Autodesk Fusion 360 part; units mm, degrees
sketch "Sketch1" plane through (0, 0, 0) normal (0, 1, 0) x (1, 0, 0) in component "SwitchSpacer"
  arc A0 (-5.8311, -8.732) -> (-5.8573, 8.7145) centre (0, 0) cw
  arc A1 (-4.6183, -9.4298) -> (-5.8311, -8.732) centre (-5.2363, -9.1011) cw
  line L0 (-20, 3.982) -> (0, 3.982)
  arc A2 (10.4756, 0.7154) -> (10.4777, -0.6839) centre (10.5, 0.0158) cw
  arc A3 (-4.6466, 9.4159) -> (10.4756, 0.7154) centre (0, 0) cw
  arc A4 (10.4777, -0.6839) -> (-4.6183, -9.4298) centre (0, 0) cw
  arc A5 (-5.8573, 8.7145) -> (-4.6466, 9.4159) centre (-5.2637, 9.0854) cw
  line L1 (-20, -4.0237) -> (-20, 3.982)
  circle A6 centre (0, 0) radius 8
  line L2 (0, 3.982) -> (0, -4.0237)
  line L3 (0, -4.0237) -> (-20, -4.0237)
  circle A7 centre (0, 0) radius 5
  circle A8 centre (0, 0) radius 4
  dimension "d8" = 10
  dimension "d9" = 8
extrude "Extrude8" add sketch "Sketch1" along normal blind 27 contours A0 A1 L0 A2 A3 A4 A5 A6 L3 | A0 L0 A6 L3 | L0 A6 L3 A7 | L0 A6 L3 A7 | L0 L2 L3 A7 A8 | L0 L2 L3 A7 A8 in component "SwitchSpacer"
sketch "Sketch2" plane through (0, 27, 0) normal (0, 1, 0) x (-1, 0, 0) in component "SwitchSpacer"
  circle A0 centre (0, 0) radius 4
  line L0 (6.35, 6.35) -> (-6.35, 6.35)
  line L1 (-6.35, 6.35) -> (-6.35, -6.35)
  line L2 (-6.35, -6.35) -> (6.35, -6.35)
  line L3 (6.35, -6.35) -> (6.35, 6.35)
  line L4 (6.35, 6.35) -> (-6.35, -6.35) construction
  line L5 (-6.35, 6.35) -> (6.35, -6.35) construction
  line L6 (6.35, 6.35) -> (19.35, 6.35)
  line L7 (19.35, 6.35) -> (19.35, -6.35)
  line L8 (19.35, -6.35) -> (6.35, -6.35)
  line L9 (6.35, -6.35) -> (6.35, 6.35)
  circle A1 centre (0, 0) radius 6.35
  line L10 (12.5, -3.5) -> (-12.5, -3.5)
  line L11 (-12.5, -3.5) -> (-12.5, 3.5)
  line L12 (-12.5, 3.5) -> (12.5, 3.5)
  line L13 (12.5, 3.5) -> (12.5, -3.5)
  line L14 (12.5, -3.5) -> (-12.5, 3.5) construction
  line L15 (-12.5, -3.5) -> (12.5, 3.5) construction
  arc A2 (5.8573, -8.7145) -> (5.8311, 8.732) centre (0, 0) ccw
  arc A3 (5.8311, 8.732) -> (4.6183, 9.4298) centre (5.2363, 9.1011) ccw
  arc A4 (4.6183, 9.4298) -> (-10.4777, 0.6839) centre (0, 0) ccw
  arc A5 (-10.4777, 0.6839) -> (-10.4756, -0.7154) centre (-10.5, -0.0158) ccw
  arc A6 (-10.4756, -0.7154) -> (4.6466, -9.4159) centre (0, 0) ccw
  arc A7 (4.6466, -9.4159) -> (5.8573, -8.7145) centre (5.2637, -9.0854) ccw
  circle A8 centre (0, 0) radius 4
  dimension "d18" = 12.7
  dimension "d19" = 12.7
  dimension "d20" = 13
  dimension "d21" = 12.7
  dimension "d22" = 12.7
  dimension "d27" = 25
  dimension "d28" = 7
extrude "Extrude9" cut sketch "Sketch1" along normal blind 6 contours L0 L2 L3 A7 A8 | L0 L2 L3 A7 A8 in component "SwitchSpacer"
extrude "Extrude10" add sketch "Sketch2" along normal blind 10 contours L0 L1 L6 L12 A2 A3 A4 | L3 L6 L9 L12 A2 | L1 L2 L8 L10 A2 A6 A7 | L3 L8 L9 L10 A2 | L1 L10 L12 A4 A5 A6 in component "SwitchSpacer"
extrude "Extrude11" cut sketch "Sketch2" against normal blind 17 contours A0 A1 L10 L12 A8 | A0 A1 L12 A8 | A0 A1 L10 A8 | A0 A1 L10 L12 A8 | L3 L9 A1 L12 | L3 L9 A1 L10 | L3 L9 L10 L12 A2 in component "SwitchSpacer"
fillet "Fillet1" radius 3 2 edges at (-7.5989, 10, -3.5) (-7.5989, 10, 3.5) in component "SwitchSpacer"
chamfer "Chamfer1" distance 0.5 angle 45 5 edges at (-6.35, 37, -4.925) (0, 37, -6.35) (-6.35, 37, 4.925) (0, 37, 6.35) (6.35, 37, 0) in component "SwitchSpacer"
component "SwitchSpacer" placed x (1, 0, 0) y (0, 1, 0) z (0, 0, 1) at (0, 0, 0)
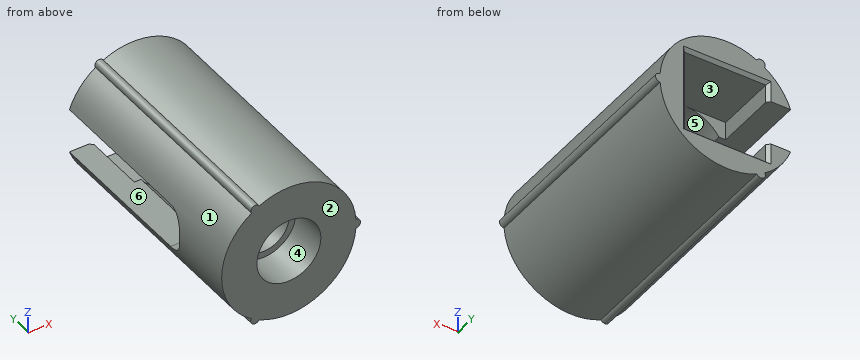
For this review, take the finished solid that the model builds, in its own axes (mm). Face numbers are marked on the shaded views. A direction names the side the tool comes from. Round coordinates to 2 decimals unless told otherwise and drop trailing zeros. Loops run counter-clockwise (first coordinate to the right, second up) from the corner with the lowest first, then second, coordinate; pieces in that order, holes last. Notation, with made-up numbers: (-20, 3.5) - (-6, 3.5) arc R30 ccw to (-6, 25.5) - close; hole circle Ø11 at (-8.75, 62.5). An arc over 180 degrees is marked (long way). Put each result on its own line as item: value. Start each with the question number.
1. For the marked faces 4, 5 and 6, list the 3-axis set-ups (+Z, -Z, +X, -X, +Y, -Y) from which the entire face can be reached by the end or side of a thin tool; tool diameter is ignored.
2. Mouldability with a two-part tool opening along X and no side actions: class the marked faces 1, 2 and 3 as +X half, -X half, draft (parallel to the pull), parting line (faces both ways), or undercut.
3. Consider section B-B on y = 7. State the section outline as (x, z) points.
4. Consider section C-C on x = -8. State the section outline as (y, z) points.
5. For probe 1 along X at (y, z) = (3.4, 0); probe 2 along X at (y, z) = (20, 0); probe 3 along Y at (x, z) = (-5.5, -2), list the stretches that pass through material, from the lowest coordinate up. Write a range as [from, to].
6. Consider section D-D on y = 16. State the section outline as (x, z) points, plus the area to 3 significant figures.
7. Insertion check: P1, Ø3, axis at x = 4, z = -3.5, coming from the +Y side; P2, Ø1, axis at y = 31.5, z = -7, coming from the +X side; P3, Ø2.5, axis at x = -7, y = 22, coming from the -Z side; P4, Ø7, axis at x = 0, z = 0, coming from the +Y side. Each pin has a flat end and moves straight along its axis. Give the tip position at first contact, or say it passes through.
8. Consider section A-A on x = -3.25. State the section outline as (y, z) points, plus the area to 3 significant figures.
Result sheet:
1. face 4: -Y
1. face 5: +Y
1. face 6: -X, +Y
2. face 1: -X half
2. face 2: draft
2. face 3: undercut
3. outline: (-5.86, -8.71) arc R0.7 ccw (long way) to (-4.65, -9.42) arc R10.5 ccw to (10.48, -0.72) arc R0.7 ccw (long way) to (10.48, 0.68) arc R10.5 ccw to (-4.62, 9.43) arc R0.7 ccw (long way) to (-5.83, 8.73) arc R10.5 ccw to start; hole circle Ø8 at (0, 0)
4. outline: (0, -6.8) - (37, -6.8) - (37, -3.5) - (13, -3.5) arc R3 cw to (10, -0.5) - (10, 0.5) arc R3 cw to (13, 3.5) - (37, 3.5) - (37, 6.8) - (0, 6.8) - close
5. probe 1: [-10.5, -5], [5, 11.2]
5. probe 2: [6.35, 11.2]
5. probe 3: [0, 10]
6. outline: (-9.9, -3.5) arc R10.5 ccw to (-5.86, -8.71) arc R0.7 ccw (long way) to (-4.65, -9.42) arc R10.5 ccw to (10.48, -0.72) arc R0.7 ccw (long way) to (10.48, 0.68) arc R10.5 ccw to (-4.62, 9.43) arc R0.7 ccw (long way) to (-5.83, 8.73) arc R10.5 ccw to (-9.9, 3.5) - (-5.3, 3.5) arc R6.35 cw (long way) to (-5.3, -3.5) - close
6. area: 192 mm^2
7. P1: y = 27
7. P2: x = 8.25
7. P3: z = -9.59
7. P4: through
8. outline: (0, -9.98) - (37, -9.98) - (37, -6.85) - (36.5, -6.35) - (27, -6.35) - (27, -5.46) - (10, -5.46) - (10, -2.33) - (6, -2.33) - (6, -3.8) - (0, -3.8) - close; (0, 3.8) - (6, 3.8) - (6, 2.33) - (10, 2.33) - (10, 5.46) - (27, 5.46) - (27, 6.35) - (36.5, 6.35) - (37, 6.85) - (37, 9.98) - (0, 9.98) - close
8. area: 362 mm^2
